Geometry: see drawing. Coordinates: mm, zero at the bounding-box minimum. A direction names the side the tool comes from. Coordinates: 2 decimals unless noted, no trailing zeros. Loops run counter-clockwise (first coordinate to the right, second up) from the corner with the lowest first, then second, coordinate; pieces in that order, holes last. Notation, with made-up numbers: (79, 36.25) -> (107, 36.25) arc R30 cw to (107, 67.25) -> close; hole circle Ø10 at (88.5, 77). An arc over 180 degrees is marked (long way). One line per item, written item: value. Start each with the question number.
Item 1: Section query C-C on z = 9.5. Return loops of the section in (x, y).
Item 2: Ray query, probe 1 along Z at (x, y) = (4.5, 25); probe 2 along Z at (x, y) = (15.75, 45.5); probe 3 along Y at (x, z) = (12, 8). Return the intervals inside material, ascending. Write a range as from..to.
Item 3: Section query A-A on y = 15.75. Return loops of the section in (x, z).
Item 4: Set-up query: the marked faces 1, 2 and 3. Return all of +Z, -Z, +X, -X, +Y, -Y with unobstructed straight access to the full face (end or side cutting, diameter ignored); none if empty.
Item 5: Section query D-D on x = 20.5. Return loops of the section in (y, z).
Item 6: Section query B-B on x = 14.5. Return loops of the section in (y, z), then the cut area to 3 significant figures.
Item 7: Contact query for flat-ended pins moving along their axis: pin 1 Ø12 at (x, y) = (4.5, 40.5) entering from +Z; pin 2 Ø6 at (x, z) = (20.5, 96) entering from -Y; pin 3 Ø3 at (x, z) = (4.5, 103.5) entering from +Y. Output: stop coordinate, or through.
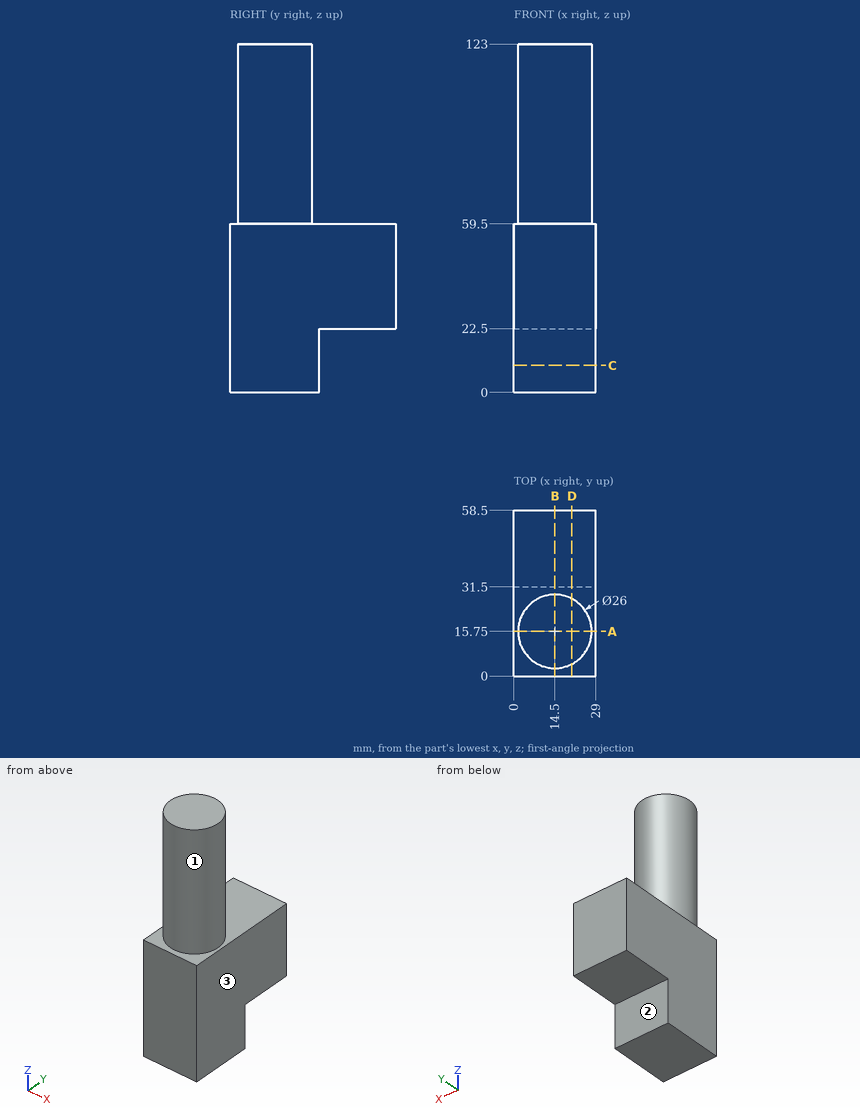
Reply:
1. outline: (0, 0) -> (29, 0) -> (29, 31.5) -> (0, 31.5) -> close
2. probe 1: z = 0..59.5
2. probe 2: z = 22.5..59.5
2. probe 3: y = 0..31.5
3. outline: (0, 0) -> (29, 0) -> (29, 59.5) -> (27.5, 59.5) -> (27.5, 123) -> (1.5, 123) -> (1.5, 59.5) -> (0, 59.5) -> close
4. face 1: +Z
4. face 2: -Z, +X, -X, +Y
4. face 3: +Z, -Z, +X, +Y, -Y
5. outline: (0, 0) -> (31.5, 0) -> (31.5, 22.5) -> (58.5, 22.5) -> (58.5, 59.5) -> (27.28, 59.5) -> (27.28, 123) -> (4.22, 123) -> (4.22, 59.5) -> (0, 59.5) -> close
6. outline: (0, 0) -> (31.5, 0) -> (31.5, 22.5) -> (58.5, 22.5) -> (58.5, 59.5) -> (28.75, 59.5) -> (28.75, 123) -> (2.75, 123) -> (2.75, 59.5) -> (0, 59.5) -> close
6. area: 4,520 mm²
7. pin 1: stops at z = 59.5
7. pin 2: stops at y = 3.1
7. pin 3: stops at y = 25.59
